The model under review builds one solid part; all positions refer to its coordinate system, in mm. Give positions to 0.01 mm unless a question says otherwise; leave off trailing zeros. Order: outer loops, then holes, each group sorted by start corner. A loop starts at its lowest first (then second) coordinate and runs counter-clockwise, first axis right, second up. Notation, with made-up numbers: (18, -8) - (22, -8) arc R29 cw to (22, 30) - close; hole circle Ø7 at (51.5, 9.5). An arc over 180 degrees is marked (long way). Write item = value, one per line. Start each with the question number.
1. For P1, Ø0.5, axis at y = 103, z = 0.5, coming from the -X side, flat-tipped, find the tip position at first contact; note if it passes through.
2. Wall thickness on probe 1 along Y at (x, z) = (14.5, 0.4); probe 2 along X at (y, z) = (83, 0.55): over which ranges is each line inside the solid? List them lowest first.
3. We need section A-A, the plane y = 43.5. Give the boundary of the cut face in (x, z), and give its area (3 significant figures).
from build123d import *

# Parameters (mm, degrees)
SKETCH1_W           = 152.4
SKETCH1_H           = 152.4
SKETCH1_W_2         = 127
SKETCH1_H_2         = 127
SKETCH1_W_3         = 18.288
SKETCH1_H_3         = 1.016
SKETCH1_W_4         = 2.032
SKETCH1_H_4         = 18.288
SKETCH1_W_5         = 1.016
SKETCH1_H_5         = 1.415312077
BOSS_EXTRUDE1_DEPTH = 1.016


with BuildPart() as part:
    # Sketch1 → Boss-Extrude1 (new body)
    # profile 1 of 22: a face of its own
    with BuildSketch(Plane.XY):
        with Locations((-7.216666869, 26.486776145)):
            Rectangle(SKETCH1_W, SKETCH1_H)
        with Locations((-7.216666869, 26.486776145)):
            Rectangle(SKETCH1_W_2, SKETCH1_H_2, mode=Mode.SUBTRACT)
    # profile 2 of 22: a face of its own
    with BuildSketch(Plane.XY):
        with Locations((59.839333131, 103.194776145)):
            Rectangle(SKETCH1_W_3, SKETCH1_H_3)
    # profile 3 of 22: a face of its own
    with BuildSketch(Plane.XY):
        with Locations((69.999333131, 93.542776145)):
            Rectangle(SKETCH1_W_4, SKETCH1_H_4)
    # profile 4 of 22: a face of its own
    with BuildSketch(Plane.XY):
        with Locations((26.311333131, 103.194776145)):
            Rectangle(SKETCH1_W_3, SKETCH1_H_3)
    # profile 5 of 22: a face of its own
    with BuildSketch(Plane.XY):
        with Locations((-7.216666869, 103.194776145)):
            Rectangle(SKETCH1_W_3, SKETCH1_H_3)
    # profile 6 of 22: a face of its own
    with BuildSketch(Plane.XY):
        with Locations((-40.744666869, 103.194776145)):
            Rectangle(SKETCH1_W_3, SKETCH1_H_3)
    # profile 7 of 22: a face of its own
    with BuildSketch(Plane.XY):
        with Locations((-74.272666869, 103.194776145)):
            Rectangle(SKETCH1_W_3, SKETCH1_H_3)
    # profile 8 of 22: a face of its own
    with BuildSketch(Plane.XY):
        with Locations((-83.924666869, 93.542776145)):
            Rectangle(SKETCH1_W_5, SKETCH1_H_4)
    # profile 9 of 22: a face of its own
    with BuildSketch(Plane.XY):
        with Locations((-83.924666869, 60.014776145)):
            Rectangle(SKETCH1_W_5, SKETCH1_H_4)
    # profile 10 of 22: a face of its own
    with BuildSketch(Plane.XY):
        with Locations((-83.924666869, -40.569223855)):
            Rectangle(SKETCH1_W_5, SKETCH1_H_4)
    # profile 11 of 22: a face of its own
    with BuildSketch(Plane.XY):
        with Locations((-74.272666869, -50.420879894)):
            Rectangle(SKETCH1_W_3, SKETCH1_H_5)
    # profile 12 of 22: a face of its own
    with BuildSketch(Plane.XY):
        with Locations((-40.744666869, -50.420879894)):
            Rectangle(SKETCH1_W_3, SKETCH1_H_5)
    # profile 13 of 22: a face of its own
    with BuildSketch(Plane.XY):
        with Locations((26.311333131, -50.420879894)):
            Rectangle(SKETCH1_W_3, SKETCH1_H_5)
    # profile 14 of 22: a face of its own
    with BuildSketch(Plane.XY):
        with Locations((-7.216666869, -50.420879894)):
            Rectangle(SKETCH1_W_3, SKETCH1_H_5)
    # profile 15 of 22: a face of its own
    with BuildSketch(Plane.XY):
        with Locations((59.839333131, -50.420879894)):
            Rectangle(SKETCH1_W_3, SKETCH1_H_5)
    # profile 16 of 22: a face of its own
    with BuildSketch(Plane.XY):
        with Locations((69.999333131, -40.569223855)):
            Rectangle(SKETCH1_W_4, SKETCH1_H_4)
    # profile 17 of 22: a face of its own
    with BuildSketch(Plane.XY):
        with Locations((69.999333131, -7.041223855)):
            Rectangle(SKETCH1_W_4, SKETCH1_H_4)
    # profile 18 of 22: a face of its own
    with BuildSketch(Plane.XY):
        with Locations((69.999333131, 26.486776145)):
            Rectangle(SKETCH1_W_4, SKETCH1_H_4)
    # profile 19 of 22: a face of its own
    with BuildSketch(Plane.XY):
        with Locations((69.999333131, 60.014776145)):
            Rectangle(SKETCH1_W_4, SKETCH1_H_4)
    # profile 20 of 22: a face of its own
    with BuildSketch(Plane.XY):
        with Locations((-7.216666869, 26.486776145)):
            Rectangle(SKETCH1_W_2, SKETCH1_H_2)
    # profile 21 of 22: a face of its own
    with BuildSketch(Plane.XY):
        with Locations((-83.924666869, 26.486776145)):
            Rectangle(SKETCH1_W_5, SKETCH1_H_4)
    # profile 22 of 22: a face of its own
    with BuildSketch(Plane.XY):
        with Locations((-83.924666869, -7.041223855)):
            Rectangle(SKETCH1_W_5, SKETCH1_H_4)
    extrude(amount=BOSS_EXTRUDE1_DEPTH)


solid = part.part
Model answer:
q1.P1 = -83.42
q2.probe_1 = -49.71 to 102.69
q2.probe_2 = -83.42 to 68.98
q3.outline = (-83.42, 0) - (68.98, 0) - (68.98, 1.02) - (-83.42, 1.02) - close
q3.area = 155 mm2
